from build123d import *

# Parameters (mm, degrees)
F1_DEPTH = 63.5
F2_DEPTH = 7.9375
F0_W     = 25.4
F0_H     = 19.05
F3_DEPTH = 25.4
F5_R     = 6.35


with BuildPart() as f1:
    # F0 (on Front) → F1 (new body, symmetric)
    with BuildSketch(Plane.XZ):
        Polygon((41.275, -9.525), (41.275, 9.525), (22.225, 9.525), (-41.275, 9.525), (-41.275, -9.525), align=None)
    extrude(amount=F1_DEPTH, both=True)

    # F0 (on Front) → F2 (join, symmetric)
    with BuildSketch(Plane.XZ):
        with BuildLine():
            Line((-41.275, 9.525), (22.225, 9.525))
            Line((22.225, 9.525), (22.225, 27.0002))
            ThreePointArc((22.225, 27.0002), (32.4542956671, 51.6959043329), (57.15, 61.9252))
            add(Edge.make_bspline(
                [(-41.275, 9.525), (-41.1499068141, 37.8207266331), (14.1535438597, 63.0222931504), (57.15, 61.9252)],
                knots=[0, 0, 0, 0, 111.5045361635, 111.5045361635, 111.5045361635, 111.5045361635], degree=3))
        make_face()
    extrude(amount=F2_DEPTH, both=True)

    # F0 (on Front) → F3 (join, symmetric)
    with BuildSketch(Plane.XZ):
        with BuildLine():
            Line((22.225, 9.525), (41.275, 9.525))
            Line((41.275, 9.525), (41.275, 27.0002))
            ThreePointArc((41.275, 27.0002), (45.9246798487, 38.2255201513), (57.15, 42.8752))
            Line((57.15, 42.8752), (60.325, 42.8752))
            Line((60.325, 42.8752), (60.325, 61.9252))
            Line((60.325, 61.9252), (57.15, 61.9252))
            ThreePointArc((57.15, 61.9252), (32.4542956671, 51.6959043329), (22.225, 27.0002))
            Line((22.225, 27.0002), (22.225, 9.525))
        make_face()
        with Locations((73.025, 52.4002)):
            Rectangle(F0_W, F0_H)
    extrude(amount=F3_DEPTH, both=True)

    # F0 (on Front) → F4 (revolve)
    with BuildSketch(Plane.XZ):
        Polygon((85.725, 61.9252), (85.725, 42.8752), (85.725, 38.1), (111.125, 38.1), (111.125, 66.675), (85.725, 66.675), align=None)
    revolve(axis=Axis((85.725, 0, 52.3875), (0, 0, -1)))

    # F5
    f5_edges = [f1.edges().sort_by_distance(p)[0] for p in [
        (-41.275, -63.5, 0),
        (41.275, -63.5, 0),
        (-41.275, 63.5, 0),
        (41.275, 63.5, 0),
    ]]
    fillet(f5_edges, radius=F5_R)


solid = f1.part
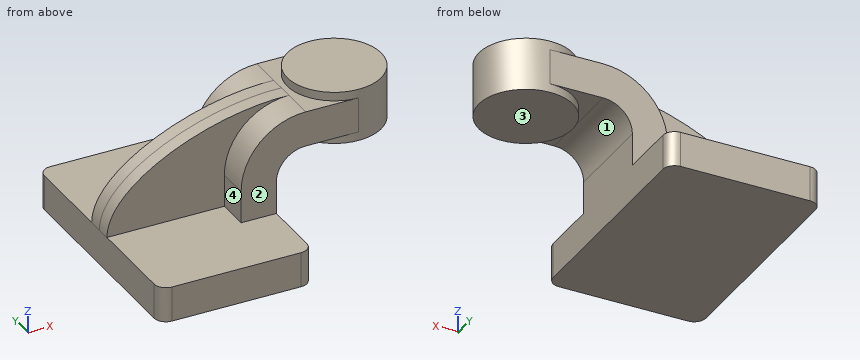
Design review of the part built by this model. Coordinates are the model's own, in mm. Face numbers are marked on the shaded views. A direction names the side the tool comes from. Round coordinates to 2 decimals unless told otherwise and drop trailing zeros. Loops run counter-clockwise (first coordinate to the right, second up) from the corner with the lowest first, then second, coordinate; pieces in that order, holes last. Notation, with made-up numbers: (88.5, 26.5) -> (113.5, 26.5) arc R17 ccw to (113.5, 50.5) -> close; hole circle Ø10 at (21.5, 53). An arc over 180 degrees is marked (long way). Use one line per item in the form item = value. Start each with the question number.
Q1. We need section D-D on y = -41. Give the boundary of the cut face in (x, z) (3 decimals).
Q2. Wall thickness on line 1 along Y through (x, z) = (64.5, 51); line 2 along Y through (x, z) = (-21, 37.5); line 3 along X through (y, z) = (-36, -1.5) (3 decimals): over which ranges is each line inside the solid? List them lowest first. Write a range as [from, to].
Q3. We need section A-A on z = -4. Give the boundary of the cut face in (x, y) (3 decimals), then the cut area to 3 significant figures.
Q4. For pin 1 Ø11 at (y, z) = (-12.5, 15) entering from +X (3 decimals); pin 2 Ø5 at (y, z) = (-18, 15) entering from -X (3 decimals); pin 3 Ø1 at (x, y) = (10.5, 46.5) entering from +Z (3 decimals), all flat-tipped, find the tip position at first contact; note any pin that passes through.
Q5. Machinability: for the marked faces 1, 2, 3 and 4, which of the approach directions +Z, -Z, +X, -X, +Y, -Y give a long, thin tool a straight path to every point of the face, cutting with its end or side? Answer none if there is none.
Q6. We need section C-C on x = 97. Give the boundary of the cut face in (y, z) (3 decimals), then the cut area to 3 significant figures.
Q7. We need section B-B on y = -18.5. Give the boundary of the cut face in (x, z) (3 decimals).
Calculated:
q1.outline = (-41.275, -9.525) -> (41.275, -9.525) -> (41.275, 9.525) -> (-41.275, 9.525) -> close
q2.line_1 = [-25.4, 25.4]
q2.line_2 = [-7.94, 7.94]
q2.line_3 = [-41.275, 41.275]
q3.outline = (-41.275, -57.15) arc R6.35 ccw to (-34.925, -63.5) -> (34.925, -63.5) arc R6.35 ccw to (41.275, -57.15) -> (41.275, 57.15) arc R6.35 ccw to (34.925, 63.5) -> (-34.925, 63.5) arc R6.35 ccw to (-41.275, 57.15) -> close
q3.area = 10,400 mm²
q4.pin_1 = 41.275
q4.pin_2 = 22.225
q4.pin_3 = 9.525
q5.face_1 = -Z, +Y, -Y
q5.face_2 = +Z, +X, -X, -Y
q5.face_3 = -Z, +X, +Y, -Y
q5.face_4 = +Z, -X, -Y
q6.outline = (-22.76, 38.1) -> (22.76, 38.1) -> (22.76, 66.675) -> (-22.76, 66.675) -> close
q6.area = 1,300 mm²
q7.outline = (-41.275, -9.525) -> (41.275, -9.525) -> (41.275, 27) arc R15.875 cw to (57.15, 42.875) -> (68.321, 42.875) -> (68.321, 38.1) -> (103.129, 38.1) -> (103.129, 66.675) -> (68.321, 66.675) -> (68.321, 61.925) -> (57.15, 61.925) arc R34.925 ccw to (22.225, 27) -> (22.225, 9.525) -> (-41.275, 9.525) -> close
